Verification items for the finished model (mm, model axes). Face numbers are marked on the shaded views. A direction names the side the tool comes from. Give positions to 0.01 mm unless a question says otherwise; leave off trailing zeros. Order: outer loops, then holes, each group sorted by start corner. A loop starts at its lowest first (then second) coordinate and runs counter-clockwise, first axis right, second up.
(1) Access from +Z, -Z, +X, -X, +Y, -Y to the whole of each face (thin tool, end or side, straight path). Record for the marked faces 4, 5, 6 and 7.
(2) Sectioned sample at A-A on y = 3.25. Record the cut outline in (x, z), plus the area to 3 significant figures.
(3) Sectioned sample at D-D on z = -6.75. Record the cut outline in (x, y), plus the area to 3 significant figures.
(4) Scan lines: L1, parallel to X at y = -0.75, z = 7; L2, parallel to Z at x = 0, y = 2.5; L3, parallel to Z at x = 9, y = -2. Record each from-to range of solid material in increasing order.
(5) Sectioned sample at B-B on y = -2.5. Record the cut outline in (x, z), plus the area to 3 significant figures.
(6) Mould release check, pull along X, two halves, no side actions. Record for the marked faces 1, 2 and 3: pulls with the +X half, pulls with the -X half, needs draft (parallel to the pull), parting line crosses it, or undercut.
(7) Gauge pin test, flat ends, axial feed: pin 1 (1.2 mm diameter, centred on x = 10, z = 7.5, fed in from -Y); pin 2 (1.4 mm diameter, centred on y = -4.5, z = -6.5, fed in from -X); pin 3 (8 mm diameter, centred on x = 10, z = 0.5, fed in from +Y). Record the tip position at first contact, or that the pin passes through.
(8) Sectioned sample at C-C on x = -6. Record the cut outline in (y, z).
```python
from build123d import *

# Parameters (mm, degrees)
SKETCH1_W           = 30.5
SKETCH1_H           = 16
BOSS_EXTRUDE1_DEPTH = 2
SKETCH3_R           = 1
SKETCH3_W           = 2.9
SKETCH3_H           = 2.8
SKETCH3_W_2         = 8
SKETCH3_H_2         = 1.1
BOSS_EXTRUDE3_DEPTH = 8
CUT_EXTRUDE2_DEPTH  = 10
CUT_EXTRUDE3_START  = -3
SKETCH5_R           = 1
SKETCH5_W           = 30.5
SKETCH5_H           = 1.1
CUT_EXTRUDE3_DEPTH  = 3
SKETCH6_W           = 30.5
SKETCH6_H           = 2
SKETCH6_W_2         = 24
BOSS_EXTRUDE4_DEPTH = 2


with BuildPart() as part:
    # Sketch1 → Boss-Extrude1 (new body)
    with BuildSketch(Plane(origin=(0, 0, 0), x_dir=(1, 0, 0), z_dir=(0, 1, 0))):
        Rectangle(SKETCH1_W, SKETCH1_H)
    extrude(amount=BOSS_EXTRUDE1_DEPTH)

    # Sketch3 → Boss-Extrude3 (add)
    with BuildSketch(Plane(origin=(0, 0, 0), x_dir=(1, 0, 0), z_dir=(0, 1, 0))):
        with Locations(Location((14.2, 4.8, 0), (0, 0, 270))):
            Circle(SKETCH3_R)
        with Locations((-4.25, 6.6)):
            Rectangle(SKETCH3_W, SKETCH3_H)
        with Locations((-11.25, -7.45)):
            Rectangle(SKETCH3_W_2, SKETCH3_H_2)
        with Locations((11.25, -7.45)):
            Rectangle(SKETCH3_W_2, SKETCH3_H_2)
    extrude(amount=-BOSS_EXTRUDE3_DEPTH)

    # Sketch4 → Cut-Extrude2 (cut)
    with BuildSketch(Plane(origin=(0, 0, 0), x_dir=(1, 0, 0), z_dir=(0, 1, 0))):
        Polygon((-15.25, 2.7), (-15.25, 8), (-8.75, 8), (-8.75, 2.7), (-8.75, 0.2), (-15.25, 0.2), align=None)
    extrude(amount=CUT_EXTRUDE2_DEPTH, mode=Mode.SUBTRACT)

    # Sketch5 → Cut-Extrude3 (cut)
    with BuildSketch(Plane.XZ.offset(8).offset(CUT_EXTRUDE3_START)):
        with Locations(Location((14.2, -4.8, 0), (0, 0, 90))):
            Circle(SKETCH5_R)
        with Locations((0, 7.45)):
            Rectangle(SKETCH5_W, SKETCH5_H)
    extrude(amount=CUT_EXTRUDE3_DEPTH, mode=Mode.SUBTRACT)

    # Sketch6 → Boss-Extrude4 (add)
    with BuildSketch(Plane(origin=(0, 2, 0), x_dir=(1, 0, 0), z_dir=(0, 1, 0))):
        with Locations((0, -7)):
            Rectangle(SKETCH6_W, SKETCH6_H)
        with Locations((3.25, 7)):
            Rectangle(SKETCH6_W_2, SKETCH6_H)
    extrude(amount=BOSS_EXTRUDE4_DEPTH)


solid = part.part
```
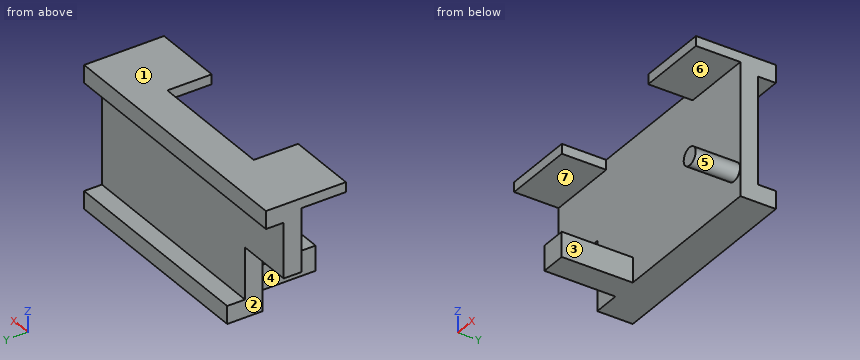
Ans:
1. face 4: +Z, -Z, -X, -Y
1. face 5: -Y
1. face 6: +X, -X, -Y
1. face 7: -Z, +X, -X, -Y
2. outline: (-15.25, 6) - (15.25, 6) - (15.25, 8) - (-15.25, 8) - close; (-8.75, -8) - (15.25, -8) - (15.25, -6) - (-8.75, -6) - close
2. area: 109 mm2
3. outline: (-8.75, 0) - (-5.7, 0) - (-5.7, -8) - (-2.8, -8) - (-2.8, 0) - (15.25, 0) - (15.25, 4) - (-8.75, 4) - close
3. area: 119 mm2
4. L1: x = -15.25 to -7.25, 7.25 to 15.25
4. L2: z = -8 to -6, 6 to 8
4. L3: z = 6.9 to 8
5. outline: (-15.25, 6.9) - (-7.25, 6.9) - (-7.25, 8) - (-15.25, 8) - close; (-5.7, -8) - (-2.8, -8) - (-2.8, -5.2) - (-5.7, -5.2) - close; (7.25, 6.9) - (15.25, 6.9) - (15.25, 8) - (7.25, 8) - close; circle Ø2 at (14.2, -4.8)
5. area: 28.9 mm2
6. face 1: needs draft
6. face 2: pulls with the -X half
6. face 3: undercut
7. pin 1: stops at y = -5
7. pin 2: stops at x = -5.7
7. pin 3: stops at y = 2
8. outline: (0, -8) - (4, -8) - (4, -6) - (2, -6) - (2, 6) - (4, 6) - (4, 8) - (0, 8) - close
